```python
from build123d import *

# Parameters (mm, degrees)
F0_R     = 60
F1_DEPTH = 10
F2_R     = 2.2
F3_DEPTH = 14
F5_DEPTH = 50
F7_DEPTH = 40
F8_R     = 4
F9_DEPTH = 10


with BuildPart() as f1:
    # F0 (on Top) → F1 (new body)
    with BuildSketch(Plane.XY):
        Circle(F0_R)
    extrude(amount=F1_DEPTH)

    # F2 (on face) → F3 (cut)
    with BuildSketch(Plane.XY.offset(10)):
        with Locations((0, 35)):
            Circle(F2_R)
        with Locations((35, 0)):
            Circle(F2_R)
        with Locations((-35, 0)):
            Circle(F2_R)
        with Locations((0, -35)):
            Circle(F2_R)
    extrude(amount=-F3_DEPTH, mode=Mode.SUBTRACT)

    # F4 (on face) → F5 (join)
    with BuildSketch(Plane.XY.offset(10)):
        with BuildLine():
            ThreePointArc((42.5, -42.5), (60.104076, 0), (42.5, 42.5))
            Line((42.5, 42.5), (42.5, -42.5))
        make_face()
        with BuildLine():
            Line((-42.5, -42.5), (-42.5, 42.5))
            ThreePointArc((-42.5, 42.5), (-60.104076, 0), (-42.5, -42.5))
        make_face()
    extrude(amount=F5_DEPTH)

    # F6 (on face) → F7 (join)
    with BuildSketch(Plane.XY.offset(60)):
        with BuildLine():
            Line((-42.5, -42.5), (-42.5, 42.5))
            ThreePointArc((-42.5, 42.5), (-47.95897, 36.227575), (-52.5, 29.26175))
            Line((-52.5, 29.26175), (-52.5, -29.26175))
            ThreePointArc((-52.5, -29.26175), (-47.95897, -36.227575), (-42.5, -42.5))
        make_face()
    extrude(amount=F7_DEPTH)

    # F8 (on face) → F9 (cut)
    with BuildSketch(Plane(origin=(-52.5, 0, 0), x_dir=(0, -1, 0), z_dir=(-1, 0, 0))):
        with Locations((0, 79.53766)):
            Circle(F8_R)
    extrude(amount=-F9_DEPTH, mode=Mode.SUBTRACT)


solid = f1.part
```
Design review of the part built by this model. Coordinates are the model's own, in mm. A direction names the side the tool comes from. Give positions to 0.01 mm unless a question says otherwise; leave off trailing zeros. Write each loop counter-clockwise with the first axis right and the second up, starting at its lowest first coordinate (ties: lowest second). Pieces come first, ordered by that corner, then holes. Notation, with made-up numbers: (-30, -15) - (-12, -15) arc R6 ccw to (-12, -9) - close; hole circle Ø10 at (59, 3.5). An arc over 180 degrees is marked (long way). Return JSON: item names as keys, results as strings. Group by question number.
(1) We need section A-A, the plane y = 0. Give the boundary of the cut face in (x, z).
(2) Insertion check: pin 1 (5 mm diameter, centred on y = 0.5, z = 77.5, fed in from -X); pin 2 (3 mm diameter, centred on y = -41, z = 52, fed in from -X); pin 3 (1 mm diameter, centred on x = -13, y = 4.5, fed in from +Z). Each pin has a flat end and moves straight along its axis. Give the tip position at first contact, or say it passes through.
(3) We need section B-B, the plane x = 0. Give the boundary of the cut face in (y, z), then the cut area to 3 significant figures.
(4) We need section D-D, the plane z = 55. Give the boundary of the cut face in (x, y).
(5) We need section C-C, the plane x = -35. Give the boundary of the cut face in (y, z).
(6) Machinability: for faces 1 (the flat face through (49, 1, 60)), 2 (the flat face through (42.5, 1, 35)), 3 (the flat face through (-52.5, 0, 75)), which of the approach directions +Z, -Z, +X, -X, +Y, -Y give a long, thin tool a straight path to every point of the face, cutting with its end or side? Answer none if there is none.
(7) Mouldability with a two-part tool opening along X and no side actions: class faces 4 (the flat face through (-42.5, -1, 54)), 5 (the flat face through (-56, 0, 60)), 6 (the cylindrical face through (-47.89, 36.32, 79.72)) as +X half, -X half, draft (parallel to the pull), parting line (faces both ways), or undercut.
(8) To check wall thickness, follow probe 1 along Y at (x, z) = (0, 4); probe 2 along Z at (x, y) = (28.5, -44.5); probe 3 along Z at (x, y) = (55.5, 15.5). State the ranges of each line that lie inside material, in increasing order.
Reported:
{
 "1": {"outline": "(-60.1, 10) - (-60, 10) - (-60, 0) - (-37.2, 0) - (-37.2, 10) - (-42.5, 10) - (-42.5, 75.54) - (-52.5, 75.54) - (-52.5, 60) - (-60.1, 60) - close; (-52.5, 83.54) - (-42.5, 83.54) - (-42.5, 100) - (-52.5, 100) - close; (-32.8, 0) - (32.8, 0) - (32.8, 10) - (-32.8, 10) - close; (37.2, 0) - (60, 0) - (60, 10) - (60.1, 10) - (60.1, 60) - (42.5, 60) - (42.5, 10) - (37.2, 10) - close"},
 "2": {"pin 1": "stops at x = -52.5", "pin 2": "stops at x = -45.3", "pin 3": "stops at z = 10"},
 "3": {"outline": "(-60, 0) - (-37.2, 0) - (-37.2, 10) - (-60, 10) - close; (-32.8, 0) - (32.8, 0) - (32.8, 10) - (-32.8, 10) - close; (37.2, 0) - (60, 0) - (60, 10) - (37.2, 10) - close", "area": "1,110 mm2"},
 "4": {"outline": "(-42.5, -42.5) - (-42.5, 42.5) arc R60.1 ccw to start; (42.5, -42.5) arc R60.1 ccw to (42.5, 42.5) - close"},
 "5": {"outline": "(-48.73, 0) - (-2.2, 0) - (-2.2, 10) - (-48.73, 10) - close; (2.2, 0) - (48.73, 0) - (48.73, 10) - (2.2, 10) - close"},
 "6": {"face 1": "+Z, +X, +Y, -Y", "face 2": "+Z, +Y, -Y", "face 3": "+Z, -X, +Y, -Y"},
 "7": {"face 4": "undercut", "face 5": "draft", "face 6": "-X half"},
 "8": {"probe 1": "y = -60 to -37.2, -32.8 to 32.8, 37.2 to 60", "probe 2": "z = 0 to 10", "probe 3": "z = 0 to 60"}
}
